The drawing under review shows one solid part. Ordinate dimensions are in mm from its lowest x, y, z. A direction names the side the tool comes from. Coordinates: 2 decimals unless noted, no trailing zeros. Loops run counter-clockwise (first coordinate to the right, second up) from the corner with the lowest first, then second, coordinate; pieces in that order, holes last. Notation, with made-up numbers: M 7,26.25 L 27,26.25 A26 cw 27,62.25 Z; hole C -28.5,60.5 d10. An arc over 180 degrees is marked long. Return JSON: item names as keys, results as strings.
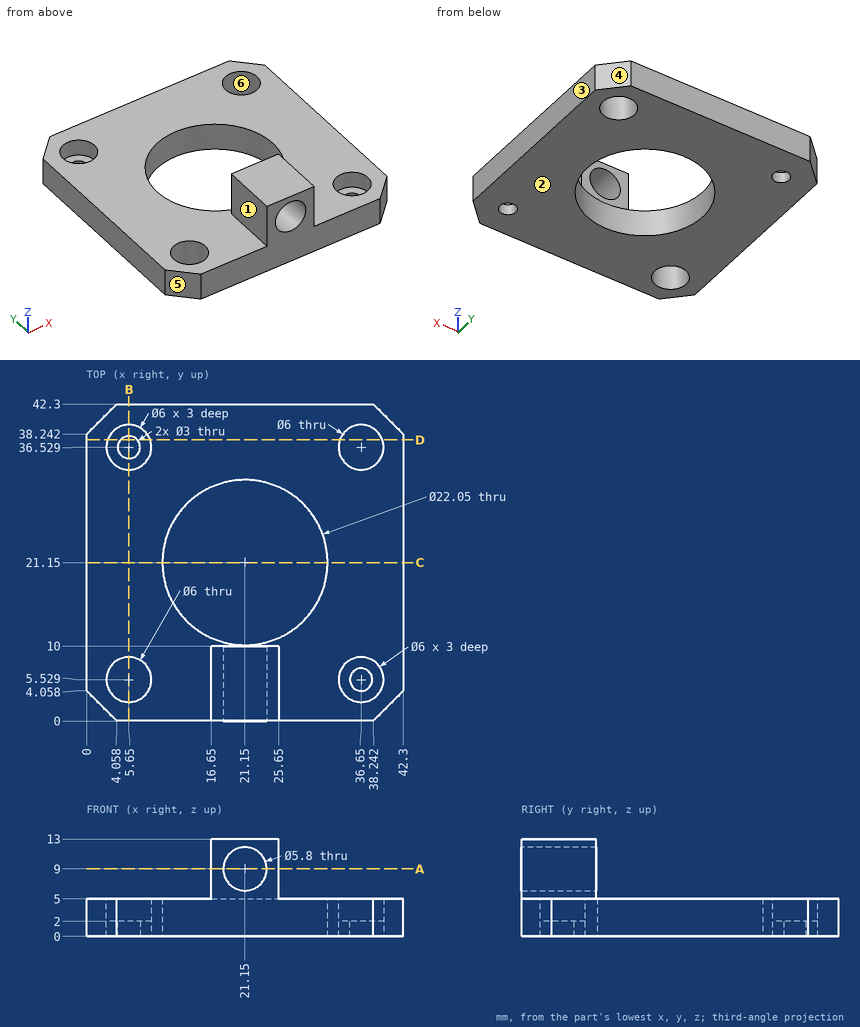
1. To check wall thickness, follow line 1 (Y direction, x = 36.65, z = 3.8); line 2 (X direction, y = 34.5, z = 3); line 3 (X direction, y = 35, z = 4.75). State the ranges of each line that lie inside material, in increasing order.
Check values:
{"line 1": "0 to 2.53, 8.53 to 33.53, 39.53 to 42.3", "line 2": "0 to 3.44, 7.86 to 34.44, 38.86 to 42.3", "line 3": "0 to 3.07, 8.23 to 34.07, 39.23 to 42.3"}
2. Add section B-B on x = 5.65. Give the boundary of the cut face in (y, z).
Check values:
{"outline": "M 0,0 L 2.53,0 L 2.53,5 L 0,5 Z; M 8.53,0 L 35.03,0 L 35.03,2 L 33.53,2 L 33.53,5 L 8.53,5 Z; M 38.03,0 L 42.3,0 L 42.3,5 L 39.53,5 L 39.53,2 L 38.03,2 Z"}
3. The part is to be moulded in two halves that separate along Y. For the marked faces 3, 4, 5 and 6, say which applies: released by +Y, released by -Y, zero draft, split by the parting line, or undercut.
Check values:
{"face 3": "zero draft", "face 4": "released by +Y", "face 5": "released by -Y", "face 6": "undercut"}
4. Insertion check: pin 1 Ø5 at (x, y) = (34.5, 27) entering from +Z; pin 2 Ø4 at (x, y) = (5.65, 36.53) entering from +Z; pin 3 Ø6.5 at (y, z) = (6.5, 9) entering from +X. Each pin has a flat end and moves straight along its axis. Give the tip position at first contact, or say it passes through.
Check values:
{"pin 1": "z = 5", "pin 2": "z = 2", "pin 3": "x = 25.65"}
5. Add section C-C on y = 21.15. Give the boundary of the cut face in (x, z) (3 decimals).
Check values:
{"outline": "M 0,0 L 10.125,0 L 10.125,5 L 0,5 Z; M 32.175,0 L 42.3,0 L 42.3,5 L 32.175,5 Z"}
6. Add section D-D on y = 37.5. Give the boundary of the cut face in (x, z).
Check values:
{"outline": "M 0,0 L 4.51,0 L 4.51,2 L 2.81,2 L 2.81,5 L 0,5 Z; M 6.79,0 L 33.81,0 L 33.81,5 L 8.49,5 L 8.49,2 L 6.79,2 Z; M 39.49,0 L 42.3,0 L 42.3,5 L 39.49,5 Z"}
7. Add section A-A on z = 9. Give the boundary of the cut face in (x, y), plus the area to 3 significant figures.
Check values:
{"outline": "M 16.65,0 L 18.25,0 L 18.25,10 L 16.65,10 Z; M 24.05,0 L 25.65,0 L 25.65,10 L 24.05,10 Z", "area": "32.0 mm²"}
8. Machinability: for the marked faces 1 and 2, which of the approach directions +Z, -Z, +X, -X, +Y, -Y give a long, thin tool a straight path to every point of the face, cutting with its end or side? Answer none if there is none.
Check values:
{"face 1": "+Z, -X, +Y, -Y", "face 2": "-Z, +X, -X, +Y, -Y"}
